For this review, use the dimensioned drawing (mm, ordinates from the lowest corner) and the shaded views. Round coordinates to 2 decimals unless told otherwise and drop trailing zeros. Loops run counter-clockwise (first coordinate to the right, second up) from the corner with the lowest first, then second, coordinate; pieces in that order, holes last. Notation, with made-up numbers: M 1,-12 L 31,-12 A14 ccw 31,8 Z; hole C -24,18 d6. An arc over 180 degrees is marked long. Answer as a JSON object with one key per item and string values. Group by question number.
Item 1: Consider section B-B (y = 148). Give the boundary of the cut face in (x, z), and give its area (3 significant figures).
Item 2: To check wall thickness, follow line 1 (X direction, y = 149.5, z = 18.5); line 2 (X direction, y = 152.5, z = 11); line 3 (Y direction, x = 10, z = 17). State the ranges of each line that lie inside material, in increasing order.
Item 3: Consider section A-A (z = 2.75). Give the boundary of the cut face in (x, y).
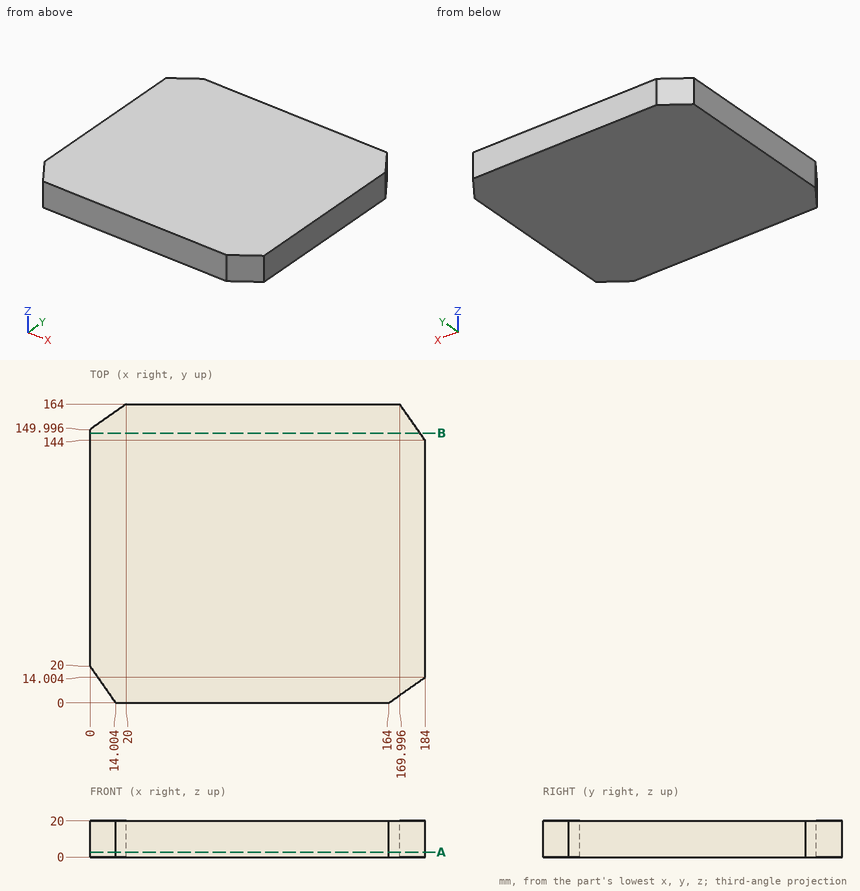
Geometry results:
{
 "1": {"outline": "M 0,0 L 181.2,0 L 181.2,20 L 0,20 Z", "area": "3,620 mm^2"},
 "2": {"line 1": "x = 0 to 180.15", "line 2": "x = 3.58 to 178.05", "line 3": "y = 5.72 to 157"},
 "3": {"outline": "M 0,20 L 14,0 L 164,0 L 184,14 L 184,144 L 170,164 L 20,164 L 0,150 Z"}
}
